from build123d import *

# Parameters (mm, degrees)
BOSS_EXTRUDE1_DEPTH = 5.08
SKETCH2_W           = 12.7
SKETCH2_H           = 5.08
CUT_EXTRUDE1_DEPTH  = 5.08


with BuildPart() as part:
    # Sketch1 → Boss-Extrude1 (new body)
    with BuildSketch(Plane.XY):
        with BuildLine():
            Line((-16.51, 12.7), (16.51, 12.7))
            Line((16.51, 12.7), (16.51, 2.54))
            ThreePointArc((16.51, 2.54), (0, -12.974722603), (-16.51, 2.54))
            Line((-16.51, 2.54), (-16.51, 12.7))
        make_face()
    extrude(amount=BOSS_EXTRUDE1_DEPTH)

    # Sketch2 → Cut-Extrude1 (cut)
    with BuildSketch(Plane.XY.offset(5.08)):
        with Locations((0, 10.16)):
            Rectangle(SKETCH2_W, SKETCH2_H)
    extrude(amount=-CUT_EXTRUDE1_DEPTH, mode=Mode.SUBTRACT)


solid = part.part
CAD build for the part. Positions are in the model's coordinates, mm. A direction names the side the tool comes from. Coordinates: 2 decimals unless noted, no trailing zeros. Loops run counter-clockwise (first coordinate to the right, second up) from the corner with the lowest first, then second, coordinate; pieces in that order, holes last. Notation, with made-up numbers: (-16, 56) - (28, 56) arc R32 cw to (28, 91) - close; hole circle Ø1 at (81.5, 35). An arc over 180 degrees is marked (long way). Write item = value, one per line. Start each with the question number.
Q1. Which spindle directions (+Z, -Z, +X, -X, +Y, -Y) get a long thin tool onto all of the face, cutting with end or side? Do faces 1 (the flat face through (6.35, 10, 3)), 2 (the flat face through (0, 0, 0)). Say none if no direction does.
Q2. Flat gauge pins, fed straight in: pin 1 Ø3 at (y, z) = (-3, 2) entering from -X; pin 2 Ø3 at (y, z) = (-8, 3.5) entering from +X; pin 3 Ø2 at (y, z) = (-3, 3.5) entering from +X. Where does each tip first touch, or does it go through?
Q3. Cut at A-A, the plane z = 4.55. List the corners of the cut face in (x, y), then the cut area to 3 significant figures.
Q4. Drill centre lines: L1, parallel to X at y = 9, z = 4.7; L2, parallel to Y at x = 7, z = 4.7; L3, parallel to Y at x = 2, z = 3.5. Where is each one in solid material? Low to high.
Q5. Cut at B-B, the plane x = 0. List the corners of the cut face in (y, z), then the cut area to 3 significant figures.
Q6. Cut at C-C, the plane y = -2. List the corners of the cut face in (x, z).
Computed:
q1.face_1 = +Z, -Z, +Y
q1.face_2 = -Z, +X, -X, +Y, -Y
q2.pin_1 = -15.75
q2.pin_2 = 13.13
q2.pin_3 = 15.58
q3.outline = (-16.51, 2.54) arc R16.54 ccw to (16.51, 2.54) - (16.51, 12.7) - (6.35, 12.7) - (6.35, 7.62) - (-6.35, 7.62) - (-6.35, 12.7) - (-16.51, 12.7) - close
q3.area = 667 mm²
q4.L1 = -16.51 to -6.35, 6.35 to 16.51
q4.L2 = -11.42 to 12.7
q4.L3 = -12.85 to 7.62
q5.outline = (-12.97, 0) - (7.62, 0) - (7.62, 5.08) - (-12.97, 5.08) - close
q5.area = 105 mm²
q6.outline = (-15.58, 0) - (15.58, 0) - (15.58, 5.08) - (-15.58, 5.08) - close
